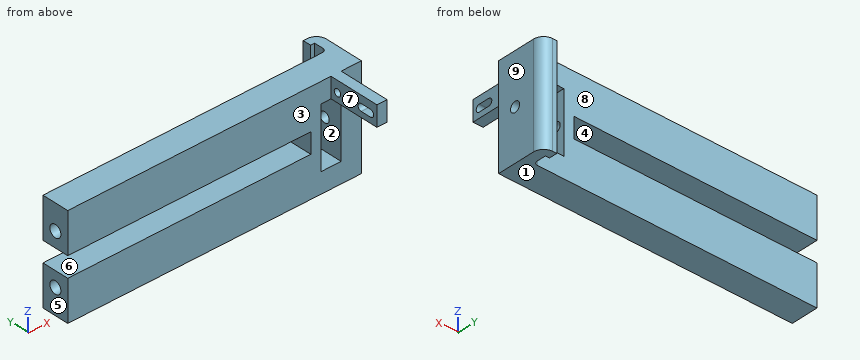
from build123d import *

# Parameters (mm, degrees)
SKETCH1_W               = 140
SKETCH1_H               = 13.5
BOSS_EXTRUDE1_DEPTH     = 50
SKETCH2_R               = 3
CUT_EXTRUDE1_DEPTH      = 5
SKETCH3_W               = 50
SKETCH3_H               = 24
BOSS_EXTRUDE2_DEPTH     = 5
CUT_EXTRUDE2_DEPTH      = 151.585523873
CUT_EXTRUDE2_DEPTH_BACK = 151.585523873
SKETCH4_W               = 10
SKETCH4_H               = 30
SKETCH5_R               = 2.5
CUT_EXTRUDE3_DEPTH      = 35
SKETCH6_W               = 50
SKETCH6_H               = 4
BOSS_EXTRUDE3_DEPTH     = 2
CUT_EXTRUDE4_DEPTH      = 150.272402004
CUT_EXTRUDE4_DEPTH_BACK = 150.272402004
SKETCH7_W               = 120
SKETCH7_H               = 10
SKETCH8_W               = 5
SKETCH8_H               = 10
BOSS_EXTRUDE4_DEPTH     = 25
CUT_EXTRUDE5_DEPTH      = 142.509716981
CUT_EXTRUDE5_DEPTH_BACK = 142.509716981
SKETCH10_R              = 1.75
FILLET1_R               = 2
FILLET2_R               = 5


with BuildPart() as part:
    # Sketch1 → Boss-Extrude1 (new body)
    with BuildSketch(Plane.XY):
        with Locations((-70, 6.75)):
            Rectangle(SKETCH1_W, SKETCH1_H)
    extrude(amount=BOSS_EXTRUDE1_DEPTH)

    # Sketch2 → Cut-Extrude1 (cut)
    with BuildSketch(Plane.ZY.offset(140)):
        with Locations((12.5, 6.75)):
            Circle(SKETCH2_R)
        with Locations((25, 6.75)):
            Circle(SKETCH2_R)
        with Locations((37.5, 6.75)):
            Circle(SKETCH2_R)
    extrude(amount=-CUT_EXTRUDE1_DEPTH, mode=Mode.SUBTRACT)

    # Sketch3 → Boss-Extrude2 (add)
    with BuildSketch(Plane(origin=(0, 0, 0), x_dir=(0, 0, -1), z_dir=(1, 0, 0))):
        with Locations((-25, 12)):
            Rectangle(SKETCH3_W, SKETCH3_H)
    extrude(amount=BOSS_EXTRUDE2_DEPTH)

    # Sketch4 → Cut-Extrude2 (cut, two sides: drawn at the far end of the back side and taken through both)
    with BuildSketch(Plane.XZ.offset(-CUT_EXTRUDE2_DEPTH_BACK)):
        with Locations((-10, 25)):
            Rectangle(SKETCH4_W, SKETCH4_H)
    extrude(amount=CUT_EXTRUDE2_DEPTH + CUT_EXTRUDE2_DEPTH_BACK, mode=Mode.SUBTRACT)

    # Sketch5 → Cut-Extrude3 (cut)
    with BuildSketch(Plane(origin=(5, 0, 0), x_dir=(0, 0, -1), z_dir=(1, 0, 0))):
        with Locations(Location((-25, 9, 0), (0, 0, 90))):
            Circle(SKETCH5_R)
    extrude(amount=-CUT_EXTRUDE3_DEPTH, mode=Mode.SUBTRACT)

    # Sketch6 → Boss-Extrude3 (add)
    with BuildSketch(Plane.ZY):
        with Locations((25, 22)):
            Rectangle(SKETCH6_W, SKETCH6_H)
    extrude(amount=BOSS_EXTRUDE3_DEPTH)

    # Sketch7 → Cut-Extrude4 (cut, two sides: drawn at the far end of the back side and taken through both)
    with BuildSketch(Plane(origin=(0, 13.5, 0), x_dir=(1, 0, 0), z_dir=(0, 1, 0)).offset(-CUT_EXTRUDE4_DEPTH_BACK)):
        with Locations((-80, -25)):
            Rectangle(SKETCH7_W, SKETCH7_H)
    extrude(amount=CUT_EXTRUDE4_DEPTH + CUT_EXTRUDE4_DEPTH_BACK, mode=Mode.SUBTRACT)

    # Sketch8 → Boss-Extrude4 (add)
    with BuildSketch(Plane.XZ):
        with Locations((-7.5, 45)):
            Rectangle(SKETCH8_W, SKETCH8_H)
    extrude(amount=BOSS_EXTRUDE4_DEPTH)

    # Sketch10 → Cut-Extrude5 (cut, two sides: drawn at the far end of the back side and taken through both)
    with BuildSketch(Plane.ZY.offset(10).offset(-CUT_EXTRUDE5_DEPTH_BACK)):
        with Locations((44.5, -3.5)):
            Circle(SKETCH10_R)
        with BuildLine():
            Line((46.25, -16.5), (46.25, -21.5))
            ThreePointArc((46.25, -21.5), (44.5, -23.25), (42.75, -21.5))
            Line((42.75, -21.5), (42.75, -16.5))
            ThreePointArc((42.75, -16.5), (44.5, -14.75), (46.25, -16.5))
        make_face()
    extrude(amount=CUT_EXTRUDE5_DEPTH + CUT_EXTRUDE5_DEPTH_BACK, mode=Mode.SUBTRACT)

    # Fillet1
    fillet1_edges = [part.edges().sort_by_distance(p)[0] for p in [
        (0, 13.5, 25),
    ]]
    fillet(fillet1_edges, radius=FILLET1_R)

    # Fillet2
    fillet2_edges = [part.edges().sort_by_distance(p)[0] for p in [
        (5, 24, 25),
    ]]
    fillet(fillet2_edges, radius=FILLET2_R)


solid = part.part
The listing builds one solid part. Answer for the finished solid, in the listing's coordinates (mm). Face numbers are marked on the shaded views. A direction names the side the tool comes from. Round coordinates to 2 decimals unless told otherwise and drop trailing zeros. Write each loop counter-clockwise with the first axis right and the second up, starting at its lowest first coordinate (ties: lowest second). Pieces come first, ordered by that corner, then holes. Notation, with made-up numbers: M 74,76 L 90,76 A14 ccw 90,103 Z; hole C -18,78.5 d6. An arc over 180 degrees is marked long. Write each question's results on one line, items separated by ' | '. Start each with the question number.
(1) Find the intervals of material crossed by line 1 (Z direction, x = -96, y = 5.5); line 2 (Z direction, x = -136, y = 6); line 3 (Z direction, x = -17.1, y = 9), in increasing order.
(2) The part is cut by section D-D, the plane y = -9.5. Write down the section's boundary in (x, z).
(3) Determine the mould class of the marked faces 1, 2, 3 and 4 for opening direction Z: +Z half, -Z half, draft (parallel to the pull), parting line (faces both ways), or undercut.
(4) For the marked faces 5, 6, 7, 8 and 9, determine the directions among +Z, -Z, +X, -X, +Y, -Y from which every point of the face is accessible in a straight line to the end or side of a thin tool.
(5) The part is cut by section B-B, the plane y = -3.5. Write down the section's boundary in (x, z).
(6) The part is cut by section A-A, the plane z = 12.5. Write down the section's boundary in (x, y).
(7) Each of these flat-tipped pins is pushed along its axis until it touches: P1, Ø12, axis at y = 4, z = 23, coming from the -X side; P2, Ø4.5, axis at y = -3.5, z = 44.5, coming from the +X side; P3, Ø2.5, axis at x = -8.5, y = -20, coming from the -Z side; P4, Ø12, axis at x = -96, z = 31, coming from the -Y side. Where does it stop, or does it pass through?
(8) The part is cut by section C-C, the plane x = -85. Write down the section's boundary in (y, z).
Worked answers:
1) line 1: z = 0 to 20, 30 to 50 | line 2: z = 0 to 9.6, 15.4 to 20, 30 to 34.6, 40.4 to 50 | line 3: z = 0 to 22.5, 27.5 to 50
2) outline: M -10,40 L -5,40 L -5,50 L -10,50 Z
3) face 1: -Z half | face 2: undercut | face 3: draft | face 4: undercut
4) face 5: +Z, -Z, -X, +Y, -Y | face 6: -X, +Y, -Y | face 7: +Z, -Z, -X, -Y | face 8: +Z, -Z, -X, +Y | face 9: +Z, -Z, +X, +Y, -Y
5) outline: M -10,40 L -5,40 L -5,42.75 L -10,42.75 Z; M -10,46.25 L -5,46.25 L -5,50 L -10,50 Z
6) outline: M -140,0 L -15,0 L -15,13.5 L -140,13.5 L -140,9.75 L -135,9.75 L -135,3.75 L -140,3.75 Z; M -5,0 L 5,0 L 5,19 A5 ccw 0,24 L -2,24 L -2,20 L 0,20 L 0,15.5 A2 cw -2,13.5 L -5,13.5 Z
7) P1: stops at x = -140 | P2: stops at x = -5 | P3: stops at z = 40 | P4: stops at y = 0
8) outline: M 0,0 L 13.5,0 L 13.5,20 L 0,20 Z; M 0,30 L 13.5,30 L 13.5,50 L 0,50 Z
